from build123d import *

# Parameters (mm, degrees)
SALIENTE_EXTRUIR1_DEPTH = 5
CROQUIS2_R              = 6
SALIENTE_EXTRUIR2_DEPTH = 8.5
CROQUIS3_R              = 4
CORTAR_EXTRUIR1_DEPTH   = 19.730545463
CHAFL_N1_SIZE           = 0.5
CROQUIS4_R              = 1.225
CORTAR_EXTRUIR2_DEPTH   = 26.294927028


with BuildPart() as part:
    # Croquis1 → Saliente-Extruir1 (new body)
    with BuildSketch(Plane.XY):
        Polygon((0, 9.814954576), (-8.5, 4.907477288), (-8.5, -4.907477288), (0, -9.814954576), (8.5, -4.907477288), (8.5, 4.907477288), align=None)
    extrude(amount=SALIENTE_EXTRUIR1_DEPTH)

    # Croquis2 → Saliente-Extruir2 (add)
    with BuildSketch(Plane.XY.offset(5)):
        Circle(CROQUIS2_R)
    extrude(amount=SALIENTE_EXTRUIR2_DEPTH)

    # Croquis3 → Cortar-Extruir1 (cut, through all)
    with BuildSketch(Plane.XY.offset(13.5)):
        Circle(CROQUIS3_R)
    extrude(amount=-CORTAR_EXTRUIR1_DEPTH, mode=Mode.SUBTRACT)

    # Chaflán1
    chafl_n1_edges = [part.edges().sort_by_distance(p)[0] for p in [
        (-6, 0, 13.5),
    ]]
    chamfer(chafl_n1_edges, length=CHAFL_N1_SIZE)

    # Croquis4 → Cortar-Extruir2 (cut, through all)
    with BuildSketch(Plane(origin=(4.25, 7.361215932, 0), x_dir=(0.8660254037844415, -0.4999999999999951, 0), z_dir=(0.49999999999999517, 0.8660254037844416, 0))):
        with Locations(Location((0, -2.5, 0), (0, 0, 180))):
            Circle(CROQUIS4_R)
    extrude(amount=-CORTAR_EXTRUIR2_DEPTH, mode=Mode.SUBTRACT)


solid = part.part
Work out the finished part from the listing and answer in its coordinate system (mm). A direction names the side the tool comes from. Round coordinates to 2 decimals unless told otherwise and drop trailing zeros. Order: outer loops, then holes, each group sorted by start corner. A loop starts at its lowest first (then second) coordinate and runs counter-clockwise, first axis right, second up. Notation, with made-up numbers: M 70,74 L 103,74 A8 ccw 103,88 Z; hole C 89.5,-8.75 d8. An arc over 180 degrees is marked long. One line per item, written item: value.
Q1. Determine the mould class of faces 3 (the face through (-8.5, 0, 2)), 4 (the face through (3.93, 4.87, 1.75)), 5 (the face through (5.254, 6.782, 1.354)) for opening direction Y: released by +Y, released by -Y, zero draft, split by the parting line, or undercut.
Derived:
face 3: zero draft
face 4: undercut
face 5: released by +Y
Q2. Find section C-C on z = 8. Write down the section's boundary in (x, y), then the cut area to 3 significant figures.
Derived:
outline: C 0,0 d12; hole C 0,0 d8
area: 62.8 mm²
Q3. For faces 1 (the face through (-4, 0, 7)), 2 (the face through (-6, 0, 9)), determine the directions among +Z, -Z, +X, -X, +Y, -Y from which every point of the face is accessible in a straight line to the end or side of a thin tool.
Derived:
face 1: +Z, -Z
face 2: +Z
Q4. Find section B-B on z = 1. Write down the section's boundary in (x, y), then the cut area to 3 significant figures.
Derived:
outline: M -8.5,-4.91 L 0,-9.81 L 8.5,-4.91 L 8.5,4.91 L 0,9.81 L -8.5,4.91 Z; hole C 0,0 d8
area: 200 mm²
Q5. Flat-ended cylindrical pins translate along their axes: pin 1 (10 mm diameter, centred on x = 0, y = -7, fed in from +Z); pin 2 (6 mm diameter, centred on y = -1.5, z = 8.5, fed in from +X); pin 3 (8 mm diameter, centred on x = -5, z = 10, fed in from -Y); pin 4 (1.5 mm diameter, centred on x = -2.5, z = 7, fed in from -Y). Find the tip coordinate at first contact, or state that the pin passes through.
Derived:
pin 1: z = 13.5
pin 2: x = 6
pin 3: y = -5.92
pin 4: y = -5.74
Q6. Straight lines are drawn through the part: line 1 (Y direction, x = 0, z = 8.25); line 2 (X direction, y = 2, z = 3); line 3 (Z direction, x = -1, y = 6). For each, find the intervals that lie inside material, in ascending order.
Derived:
line 1: -6 to -4, 4 to 6
line 2: -8.5 to -3.46, 3.46 to 8.5
line 3: 0 to 5
Q7. Find section A-A on y = 0. Write down the section's boundary in (x, z), then the cut area to 4 significant figures.
Derived:
outline: M -8.5,0 L -4,0 L -4,13.5 L -5.5,13.5 L -6,13 L -6,5 L -8.5,5 Z; M 4,0 L 8.5,0 L 8.5,5 L 6,5 L 6,13 L 5.5,13.5 L 4,13.5 Z
area: 78.75 mm²
Q8. Find section D-D on x = -7. Write down the section's boundary in (y, z), then the cut area to 3 significant figures.
Derived:
outline: M -5.77,0 L 5.77,0 L 5.77,5 L -5.77,5 Z
area: 57.7 mm²
